Can you work these out from the model? Positions are in its coordinate system, mm. Face numbers are marked on the shaded views. A direction names the side the tool comes from. Give positions to 0.01 mm unless a question says otherwise; leave off trailing zeros. Write each loop counter-clockwise with the first axis right and the second up, starting at its lowest first coordinate (ties: lowest second). Pieces come first, ordered by that corner, then holes. Notation, with made-up numbers: (21.25, 78.5) -> (53.25, 78.5) arc R15 cw to (53.25, 103.5) -> close; hole circle Ø5 at (75.25, 41.25). An arc over 180 degrees is marked (long way). One line per item, written item: value.
Autodesk Inventor part; units mm, degrees
ref_plane "XZ Plane" through (0, 0, 0) normal (0, 1, 0) x (-1, 0, 0)
ref_plane "XY Plane" through (0, 0, 0) normal (0, 0, 1) x (1, 0, 0)
sketch "Bolt sketch" plane through (0, 0, 0) normal (0, 0, 1) x (1, 0, 0)
  circle A0 centre (0, 0) radius 3.175
  dimension "d0" = 6.35
extrude "Bolt extrution" add sketch "Bolt sketch" along normal blind 25.4
thread "Axle peg Thread"
sketch "Head Sketch" plane through (0, 0, 0) normal (1, 0, 0) x (0, 1, 0)
  line L0 (3.175, 25.4) -> (-3.175, 25.4)
  line L1 (0, 25.4) -> (5.3594, 25.4)
  line L2 (5.3594, 25.4) -> (5.3594, 26.1874)
  line L3 (0, 25.4) -> (0, 28.575)
  line L4 (0, 28.575) -> (3.175, 28.575)
  arc A0 (5.3594, 26.1874) -> (3.175, 28.575) centre (0.0087, 23.4851) ccw
  point P0 (0, 0)
  dimension "d5" = 5.3594
  dimension "d6" = 0.7874
  dimension "d7" = 3.175
  dimension "d8" = 3.175
  dimension "d9" = 5.9944
revolve "Revolution1" add sketch "Head Sketch" angle 360 about axis through (0, 0, 25.4) along (0, 0, 1)
sketch "Hexagon sketch" plane through (0, 0, 28.575) normal (0, 0, 1) x (1, 0, 0)
  line L0 (1.1498, -1.9844) -> (-1.1498, -1.9844)
  line L1 (-1.1498, -1.9844) -> (-2.2873, 0)
  line L2 (-2.2873, 0) -> (-1.1498, 1.9844)
  line L3 (-1.1498, 1.9844) -> (1.1569, 1.9844)
  line L4 (1.1569, 1.9844) -> (2.2873, 0)
  line L5 (2.2873, 0) -> (1.1498, -1.9844)
  line L6 (0, 0) -> (3.4356, 0) construction
  line L7 (0, 0) -> (-2.586, 0) construction
  dimension "d13" = 3.9688
  dimension "d15" = 3.9688
  dimension "d16" = 0.156
  dimension "d17" = 1.9844
  dimension "d18" = 1.9844
  dimension "d19" = 1.9844
  dimension "d20" = 1.9875
extrude "Hexagon Hole extrution" cut sketch "Hexagon sketch" against normal blind 2.8194
chamfer "Bottom Chamfer" distance 0.762 angle 45 1 edges at (-3.175, 0, 0)
properties part number "Caufield_Axle_Peg"
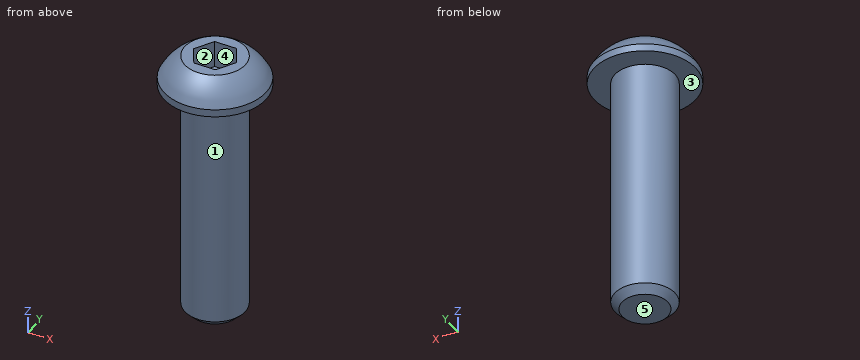
1) Will these pins go through, and if not, where does the flat tip stop? pin 1 (1 mm diameter, centred on y = 0, z = 14, fed in from -X) (3 decimals); pin 2 (1.1 mm diameter, centred on x = 0.5, z = 27, fed in from +Y); pin 3 (2 mm diameter, centred on x = 1.5, z = 23.5, fed in from +Y).
Answer list:
pin 1: stops at x = -3.175
pin 2: stops at y = 5.2
pin 3: stops at y = 3.14
2) We'd pull the mould along Y, two halves only. Please class the marked faces 1, 2 and 3: released by +Y, released by -Y, zero draft, split by the parting line, or undercut.
Answer list:
face 1: split by the parting line
face 2: undercut
face 3: zero draft
3) I need wall thicknesses on L1, parallel to Z at x = 0, y = -1.25; L2, parallel to X at y = 1, z = 5.25; L3, parallel to Z at x = 4.75, y = 1. Which ranges of each line are inside material? Lowest first, please.
Answer list:
L1: z = 0 to 25.76
L2: x = -3.01 to 3.01
L3: z = 25.4 to 27.01
4) For the marked faces 4 and 5, which set-ups out of +Z, -Z, +X, -X, +Y, -Y let a thin tool reach every point of the face, with its end or its side?
Answer list:
face 4: +Z
face 5: -Z, +X, -X, +Y, -Y
5) If we section it at A-A (z = 23.5): Write out the boundary of the cut face in (x, y) (3 decimals).
Answer list:
outline: circle Ø6.35 at (0, 0)
